Check sheet for the modelled part. Datum: model origin and axes. Units: mm. A direction names the side the tool comes from. Coordinates: 2 decimals unless noted, no trailing zeros. Order: outer loops, then holes, each group sorted by start corner. A loop starts at its lowest first (then second) coordinate and runs counter-clockwise, first axis right, second up. Notation, with made-up numbers: M 34.25,-2 L 85.25,-2 A23 ccw 85.25,12 Z; hole C 30.5,29 d2. An arc over 180 degrees is marked long. Answer in a Markdown table with one row per item. Add a question column.
from build123d import *

# Parameters (mm, degrees)
SKETCH_W     = 135
SKETCH_H     = 20
PAD_DEPTH    = 10
POCKET_DEPTH = 10


with BuildPart() as part:
    # Sketch → Pad (new body)
    with BuildSketch(Plane.XY):
        with Locations((0.531994, 1.222491)):
            Rectangle(SKETCH_W, SKETCH_H)
    extrude(amount=PAD_DEPTH)

    # Sketch001 (on Face6 of Pad) → Pocket (cut)
    with BuildSketch(Plane.XY.offset(10)):
        Polygon((-66.968006, 8.722491), (-59.218006, 4.248027), (-59.218006, 16.222491), (-71.968006, 16.222491), (-71.968006, -13.777509), (-59.218006, -13.777509), (-59.218006, -1.803044), (-66.968006, -6.277509), align=None)
        Polygon((68.031994, 8.722491), (60.281994, 4.248027), (60.281994, 16.222491), (73.031994, 16.222491), (73.031994, -13.777509), (60.281994, -13.777509), (60.281994, -1.803044), (68.031994, -6.277509), align=None)
    extrude(amount=-POCKET_DEPTH, mode=Mode.SUBTRACT)


solid = part.part
1. Set-up check for faces 1 (the flat face through (-59.218, -5, 5)), 2 (the flat face through (-63.15, 6.52, 5.07)), 3 (the flat face through (68.032, 1, 5)): record each of +Z, -Z, +X, -X, +Y, -Y from which the full face is reachable in a straight line by a thin tool's end or side.
2. Section check B-B on z = 1.25. Enter the section's corners in (x, y).
3. Scan lines: line 1 (X direction, y = 8, z = 3.5); line 2 (X direction, y = -4.25, z = 5.25); line 3 (X direction, y = 9.75, z = 4.75). Record each from-to range of solid material in increasing order.
4. Release check for a two-part mould opening along X. For faces 4 (the flat face through (-66.968, 1, 5)), 5 (the flat face through (0, 1, 10)), 6 (the flat face through (60.282, 8, 5)) record: released by +X, released by -X, zero draft, split by the parting line, or undercut.
5. Section check A-A on y = 6.25. Enter the section's corners in (x, z), then the cut area to 3 significant figures.
6. Section check C-C on y = -4.75. Enter the section's corners in (x, z), then the cut area to 3 significant figures.
Result sheet:
| question | item | result |
|---|---|---|
| 1 | face 1 | +Z, -Z, -Y |
| 1 | face 2 | +Z, -Z, +Y |
| 1 | face 3 | +Z, -Z, +X, +Y, -Y |
| 2 | outline | M -66.97,-6.28 L -59.22,-1.8 L -59.22,-8.78 L 60.28,-8.78 L 60.28,-1.8 L 68.03,-6.28 L 68.03,8.72 L 60.28,4.25 L 60.28,11.22 L -59.22,11.22 L -59.22,4.25 L -66.97,8.72 Z |
| 3 | line 1 | -66.97 to -65.72, -59.22 to 60.28, 66.78 to 68.03 |
| 3 | line 2 | -66.97 to -63.46, -59.22 to 60.28, 64.52 to 68.03 |
| 3 | line 3 | -59.22 to 60.28 |
| 4 | face 4 | released by -X |
| 4 | face 5 | zero draft |
| 4 | face 6 | undercut |
| 5 | outline | M -66.97,0 L -62.69,0 L -62.69,10 L -66.97,10 Z; M -59.22,0 L 60.28,0 L 60.28,10 L -59.22,10 Z; M 63.75,0 L 68.03,0 L 68.03,10 L 63.75,10 Z |
| 5 | area | 1,280 mm^2 |
| 6 | outline | M -66.97,0 L -64.32,0 L -64.32,10 L -66.97,10 Z; M -59.22,0 L 60.28,0 L 60.28,10 L -59.22,10 Z; M 65.39,0 L 68.03,0 L 68.03,10 L 65.39,10 Z |
| 6 | area | 1,250 mm^2 |
